Geometry: final body of the model. Coordinates: model frame, mm. Coordinates: 2 decimals unless noted, no trailing zeros. Order: outer loops, then holes, each group sorted by start corner. A loop starts at its lowest first (then second) coordinate and runs counter-clockwise, first axis right, second up. Notation, with made-up numbers: M 44,-33.75 L 99,-33.75 A11 cw 99,-16.75 Z; hole C 71,-4.75 d7. An arc over 180 degrees is marked long. Use CSV: the item, a comma, the result in double quotes. Start each with the question number.
1. Pull-direction query (X, two-part tool) for faces 1 (the flat face through (118, 8, -20)), 2 (the flat face through (125, 7, -10)), 3 (the cylindrical face through (42.84, 6.54, -10.37)); classes: pulls with the +X half, pulls with the -X half, needs draft (parallel to the pull), parting line crosses it, or undercut.
2. Material intervals for line 1 (X direction, y = 7.75, z = -12.75); line 2 (Y direction, x = 40.53, z = -9); line 3 (X direction, y = 11.5, z = -15), sorted ascending.
3. Section query C-C on y = 2.25. Return the cut outline in (x, z), and give its area (3 significant figures).
4. Section query B-B on y = 7.5. Return the cut outline in (x, z), and give its area (3 significant figures).
5. Section query A-A on x = 85.03. Return the cut outline in (y, z), and give its area (3 significant figures).
6. First-contact query: P1, Ø3, axis at x = 85.5, y = 6, coming from the +Z side. Flat tip, straight axial feed; report the tip coordinate or a pass-through.
from build123d import *

# Parameters (mm, degrees)
SKETCH_1_W          = 125
SKETCH_1_H          = 40
EXTRUDE_1_DEPTH     = 15
SKETCH_2_R          = 9.1
SKETCH_2_R_2        = 4.6
SKETCH_2_R_3        = 13.3
CUT_EXTRUDE_1_DEPTH = 133.098448136
CHAMFER_1_SIZE      = 1
CHAMFER_2_SIZE      = 1
FILLET_1_R          = 1
SKETCH_3_R          = 2.5
CUT_EXTRUDE_2_DEPTH = 133.098448136
FILLET_2_R          = 1
SKETCH_5_W          = 130.4461144
SKETCH_5_H          = 31.847563365
CUT_EXTRUDE_3_DEPTH = 133.098448178


with BuildPart() as part:
    # 草圖1 → 填料-伸長1 (new body)
    with BuildSketch(Plane(origin=(0, 0, 0), x_dir=(1, 0, 0), z_dir=(0, 1, 0))):
        with Locations((62.5, 20)):
            Rectangle(SKETCH_1_W, SKETCH_1_H)
    extrude(amount=EXTRUDE_1_DEPTH)

    # 草圖2 → 除料-伸長1 (cut, through all)
    with BuildSketch(Plane(origin=(0, 15, 0), x_dir=(1, 0, 0), z_dir=(0, 1, 0))):
        with Locations(Location((18.526668527, 20, 0), (0, 0, 270))):
            Circle(SKETCH_2_R)
        with Locations(Location((107.526668527, 20, 0), (0, 0, 270))):
            Circle(SKETCH_2_R_2)
        with Locations(Location((62.526668527, 20, 0), (0, 0, 270))):
            Circle(SKETCH_2_R_3)
    extrude(amount=-CUT_EXTRUDE_1_DEPTH, mode=Mode.SUBTRACT)

    # 導角1
    chamfer_1_edges = [part.edges().sort_by_distance(p)[0] for p in [
        (18.526668527, 15, -29.1),
    ]]
    chamfer(chamfer_1_edges, length=CHAMFER_1_SIZE)

    # 導角2
    chamfer_2_edges = [part.edges().sort_by_distance(p)[0] for p in [
        (18.526668527, 0, -29.1),
    ]]
    chamfer(chamfer_2_edges, length=CHAMFER_2_SIZE)

    # 圓角1
    fillet_1_edges = [part.edges().sort_by_distance(p)[0] for p in [
        (107.526668527, 0, -24.6),
        (107.526668527, 15, -24.6),
        (62.526668527, 0, -33.3),
        (62.526668527, 15, -33.3),
    ]]
    fillet(fillet_1_edges, radius=FILLET_1_R)

    # 草圖3 → 除料-伸長2 (cut, through all)
    with BuildSketch(Plane.XY):
        with Locations((40.53, 7.5)):
            Circle(SKETCH_3_R)
        with Locations((85.03, 7.5)):
            Circle(SKETCH_3_R)
    extrude(amount=-CUT_EXTRUDE_2_DEPTH, mode=Mode.SUBTRACT)

    # 圓角2
    fillet_2_edges = [part.edges().sort_by_distance(p)[0] for p in [
        (38.03, 7.5, -40),
        (38.03, 7.5, 0),
        (82.53, 7.5, -40),
        (82.53, 7.5, 0),
    ]]
    fillet(fillet_2_edges, radius=FILLET_2_R)

    # 草圖5 → 除料-伸長3 (cut, through all)
    with BuildSketch(Plane(origin=(0, 15, 0), x_dir=(1, 0, 0), z_dir=(0, 1, 0))):
        with Locations((65.2230572, 35.923781683)):
            Rectangle(SKETCH_5_W, SKETCH_5_H)
    extrude(amount=-CUT_EXTRUDE_3_DEPTH, mode=Mode.SUBTRACT)


solid = part.part
Results list:
1,face 1,"needs draft"
1,face 2,"pulls with the +X half"
1,face 3,"undercut"
2,line 1,"x = 0 to 13.03, 24.03 to 38.04, 43.02 to 51.38, 73.68 to 82.54, 87.52 to 125"
2,line 2,"y = 0 to 5, 10 to 15"
2,line 3,"x = 0 to 10.92, 26.13 to 50.2, 74.85 to 125"
3,outline,"M 0,-20 L 9.43,-20 A9.1 cw 27.63,-20 L 49.23,-20 A13.3 cw 75.83,-20 L 102.93,-20 A4.6 cw 112.13,-20 L 125,-20 L 125,0 L 0,0 Z"
3,area,"2,060 mm²"
4,outline,"M 0,-20 L 9.43,-20 A9.1 cw 27.63,-20 L 38.03,-20 L 38.03,-1 A1 ccw 37.03,0 L 0,0 Z; M 43.03,-20 L 49.23,-20 A13.3 cw 75.83,-20 L 82.53,-20 L 82.53,-1 A1 ccw 81.53,0 L 44.03,0 A1 ccw 43.03,-1 Z; M 87.53,-20 L 102.93,-20 A4.6 cw 112.13,-20 L 125,-20 L 125,0 L 88.53,0 A1 ccw 87.53,-1 Z"
4,area,"1,860 mm²"
5,outline,"M 0,-20 L 5,-20 L 5,-1 A1 ccw 4,0 L 0,0 Z; M 10,-20 L 15,-20 L 15,0 L 11,0 A1 ccw 10,-1 Z"
5,area,"200 mm²"
6,P1,"stops at z = -0.1"
